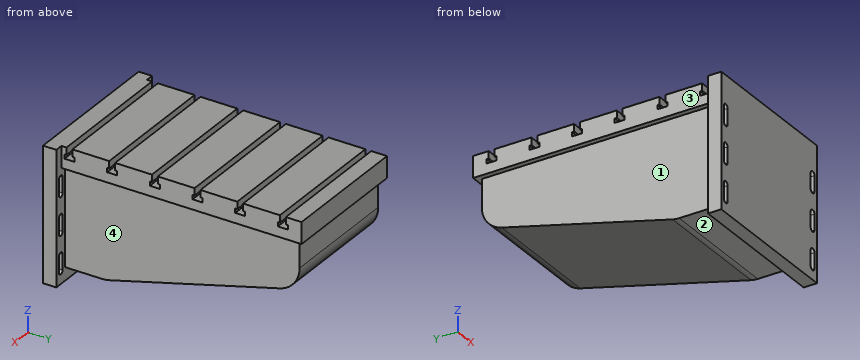
```python
from build123d import *

# Parameters (mm, degrees)
BOSS_EXTRUDE1_DEPTH  = 280
CUT_EXTRUDE2_REACH   = 1068.958
CUT_EXTRUDE3_REACH   = 1111.459
LPATTERN2_COUNT      = 3
LPATTERN2_PITCH      = 140
CUT_EXTRUDE1_REACH   = 1212.826
LPATTERN1_COUNT      = 6
LPATTERN1_PITCH      = 160
MIRROR1_COPY_1_REACH = 1111.459
MIRROR1_COPY_2_REACH = 1111.459


with BuildPart() as part:
    # Sketch4 → Boss-Extrude1 (new, symmetric)
    with BuildSketch(Plane(origin=(0, 0, 0), x_dir=(0, 0, -1), z_dir=(1, 0, 0))):
        with BuildLine():
            Line((0, 0), (0, 950))
            Line((0, 950), (80, 950))
            Line((80, 950), (80, 930))
            Line((80, 930), (182.772011822, 930))
            ThreePointArc((182.772011822, 930), (243.894588799, 909.145628961), (279.523707794, 855.280611672))
            Line((279.523707794, 855.280611672), (446.751695972, 215.280611672))
            ThreePointArc((446.751695972, 215.280611672), (449.184599604, 202.744222275), (450, 190))
            Line((450, 190), (450, 50))
            Line((450, 50), (500, 50))
            Line((500, 50), (500, 0))
            Line((500, 0), (0, 0))
        make_face()
    extrude(amount=BOSS_EXTRUDE1_DEPTH, both=True)

    # Sketch9 → Cut-Extrude2 (cut, up to next)
    with BuildSketch(Plane(origin=(0, 50, 0), x_dir=(1, 0, 0), z_dir=(0, 1, 0)), mode=Mode.PRIVATE) as cut_extrude2_sk1:
        Polygon((-230, 80), (-250, 80), (-250, -10), (-330, -10), (-330, 560), (-230, 560), align=None)
    cut_extrude2_tool1 = extrude(cut_extrude2_sk1.sketch, amount=CUT_EXTRUDE2_REACH, mode=Mode.PRIVATE) & part.part
    cut_extrude2 = cut_extrude2_tool1.solids().sort_by_distance((-281.304348, 50, -282.826087))[0]
    add(cut_extrude2, mode=Mode.SUBTRACT)

    # Sketch10 → Cut-Extrude3 (cut, up to next)
    with BuildSketch(Plane.XZ, mode=Mode.PRIVATE) as cut_extrude3_sk1:
        with BuildLine():
            Line((-243, -116), (-243, -174))
            ThreePointArc((-243, -174), (-254, -185), (-265, -174))
            Line((-265, -174), (-265, -116))
            ThreePointArc((-265, -116), (-254, -105), (-243, -116))
        make_face()
    cut_extrude3_tool1 = extrude(cut_extrude3_sk1.sketch, amount=-CUT_EXTRUDE3_REACH, mode=Mode.PRIVATE) & part.part
    cut_extrude3 = cut_extrude3_tool1.solids().sort_by_distance((-254, 0, -145))[0]
    add(cut_extrude3, mode=Mode.SUBTRACT)

    # LPattern2: Cut-Extrude3 ×3
    with Locations(*[(0, 0, -i * LPATTERN2_PITCH) for i in range(1, LPATTERN2_COUNT)]):
        add(cut_extrude3, mode=Mode.SUBTRACT)

    # Sketch6 → Cut-Extrude1 (cut, up to next)
    with BuildSketch(Plane(origin=(280, 0, 0), x_dir=(0, 0, -1), z_dir=(1, 0, 0)), mode=Mode.PRIVATE) as cut_extrude1_sk1:
        Polygon((0, 69), (0, 91), (26.9, 91), (26.9, 98.6), (43, 98.6), (43, 61.4), (26.9, 61.4), (26.9, 69), align=None)
    cut_extrude1_tool1 = extrude(cut_extrude1_sk1.sketch, amount=-CUT_EXTRUDE1_REACH, mode=Mode.PRIVATE) & part.part
    cut_extrude1 = cut_extrude1_tool1.solids().sort_by_distance((280, 80, -24.26428))[0]
    add(cut_extrude1, mode=Mode.SUBTRACT)

    # LPattern1: Cut-Extrude1 ×6
    with Locations(*[(0, i * LPATTERN1_PITCH, 0) for i in range(1, LPATTERN1_COUNT)]):
        add(cut_extrude1, mode=Mode.SUBTRACT)

    # Mirror1: Cut-Extrude2, Cut-Extrude3 across plane
    add(cut_extrude2.mirror(Plane(origin=(0, 0, 0), x_dir=(0, 0, 1), z_dir=(1, 0, 0))), mode=Mode.SUBTRACT)
    add(cut_extrude3.mirror(Plane(origin=(0, 0, 0), x_dir=(0, 0, 1), z_dir=(1, 0, 0))), mode=Mode.SUBTRACT)

    # Mirror1 copy 1 sketch → Mirror1 copy 1 (cut, up to next)
    with BuildSketch(Plane(origin=(0, 0, -140), x_dir=(-1, 0, 0), z_dir=(0, -1, 0)), mode=Mode.PRIVATE) as mirror1_copy_1_sk1:
        with BuildLine():
            Line((-243, 116), (-243, 174))
            ThreePointArc((-243, 174), (-254, 185), (-265, 174))
            Line((-265, 174), (-265, 116))
            ThreePointArc((-265, 116), (-254, 105), (-243, 116))
        make_face()
    mirror1_copy_1_tool1 = extrude(mirror1_copy_1_sk1.sketch, amount=-MIRROR1_COPY_1_REACH, mode=Mode.PRIVATE) & part.part
    add(mirror1_copy_1_tool1.solids().sort_by_distance((254, 0, -285))[0], mode=Mode.SUBTRACT)

    # Mirror1 copy 2 sketch → Mirror1 copy 2 (cut, up to next)
    with BuildSketch(Plane(origin=(0, 0, -280), x_dir=(-1, 0, 0), z_dir=(0, -1, 0)), mode=Mode.PRIVATE) as mirror1_copy_2_sk1:
        with BuildLine():
            Line((-243, 116), (-243, 174))
            ThreePointArc((-243, 174), (-254, 185), (-265, 174))
            Line((-265, 174), (-265, 116))
            ThreePointArc((-265, 116), (-254, 105), (-243, 116))
        make_face()
    mirror1_copy_2_tool1 = extrude(mirror1_copy_2_sk1.sketch, amount=-MIRROR1_COPY_2_REACH, mode=Mode.PRIVATE) & part.part
    add(mirror1_copy_2_tool1.solids().sort_by_distance((254, 0, -425))[0], mode=Mode.SUBTRACT)


solid = part.part
```
Geometry check sheet. Reference: the model listing, model coordinates, mm. Face numbers are marked on the shaded views. A direction names the side the tool comes from. Give positions to 0.01 mm unless a question says otherwise; leave off trailing zeros. Write each loop counter-clockwise with the first axis right and the second up, starting at its lowest first coordinate (ties: lowest second). Pieces come first, ordered by that corner, then holes. Notation, with made-up numbers: (25.5, 39) - (81.5, 39) arc R11 ccw to (81.5, 57) - close; hole circle Ø5 at (-18.75, 62). An arc over 180 degrees is marked (long way). Use a Markdown table: item, result.
Q1. Thickness scan on L1, parallel to Z at x = 245.5, y = 806; L2, parallel to X at y = 144, z = -162.5; L3, parallel to Z at x = 181, y = 154.5. Record the ranges inside material, lowest first. Write a range as [from, to].
Computed:
| item | result |
|---|---|
| L1 | z = [-80, 0] |
| L2 | x = [-230, 230] |
| L3 | z = [-450, 0] |
Q2. Section check B-B, the plane z = -212. Enter the section's corners in (x, y).
Computed:
| item | result |
|---|---|
| outline | (-280, 0) - (280, 0) - (280, 50) - (230, 50) - (230, 925.63) - (-230, 925.63) - (-230, 50) - (-280, 50) - close |
Q3. Section check A-A, the plane y = 147.5. Enter the section's corners in (x, z), then the cut area to 3 significant figures.
Computed:
| item | result |
|---|---|
| outline | (-250, -80) - (-230, -80) - (-230, -450) - (230, -450) - (230, -80) - (250, -80) - (250, 0) - (-250, 0) - close |
| area | 210,000 mm² |
Q4. Set-up check for the marked faces 1, 2, 3 and 4: record each of +Z, -Z, +X, -X, +Y, -Y from which the full face is reachable in a straight line by a thin tool's end or side.
Computed:
| item | result |
|---|---|
| face 1 | -Z, -X, +Y |
| face 2 | -Z, +X, -X, +Y |
| face 3 | +Z, -Z, -X, +Y |
| face 4 | -Z, +X, +Y |
Q5. Go/stop test with flat-tipped pins: P1, Ø12, axis at x = 127, y = 640.5, coming from the -Z side; P2, Ø5, axis at y = 632, z = -101, coming from the +X side; P3, Ø1, axis at y = 348, z = -234.5, coming from the -X side. Record where each tip stops, or that it passes through.
Computed:
| item | result |
|---|---|
| P1 | stops at z = -337.21 |
| P2 | stops at x = 230 |
| P3 | stops at x = -230 |
